```python
from build123d import *

# Parameters (mm, degrees)
ESQUISSE1_W        = 10
ESQUISSE1_H        = 3
ESQUISSE1_W_2      = 3
ESQUISSE1_H_2      = 10
BOSS_EXTRU_1_DEPTH = 3


with BuildPart() as part:
    # Esquisse1 → Boss.-Extru.1 (new body)
    with BuildSketch(Plane(origin=(0, 0, 0), x_dir=(1, 0, 0), z_dir=(0, 1, 0))):
        with BuildLine():
            Line((-48.586354215, -63.79082471), (72.626849221, -63.79082471))
            Line((72.626849221, -63.79082471), (72.626849221, -31.820261962))
            Line((72.626849221, -31.820261962), (61.846203207, -42.600907976))
            ThreePointArc((61.846203207, -42.600907976), (59.121902654, -51.239420877), (50.947990526, -47.336488751))
            Line((50.947990526, -47.336488751), (19.393465144, -47.336488751))
            Line((19.393465144, -47.336488751), (19.393465144, -44.336488751))
            Line((19.393465144, -44.336488751), (50.896342586, -44.336488751))
            ThreePointArc((50.896342586, -44.336488751), (54.339544234, -40.233556625), (59.688362254, -40.516108241))
            Line((59.688362254, -40.516108241), (72.626849221, -27.577621274))
            Line((72.626849221, -27.577621274), (72.626849221, -17.577621274))
            Line((72.626849221, -17.577621274), (-27.373150779, -17.577621274))
            Line((-27.373150779, -17.577621274), (-48.586354215, -38.79082471))
            Line((-48.586354215, -38.79082471), (-48.586354215, -63.79082471))
        make_face()
        with Locations((-1.907227595, -25.374770958)):
            Rectangle(ESQUISSE1_W, ESQUISSE1_H, mode=Mode.SUBTRACT)
        with Locations((-21.907227595, -25.374770958)):
            Rectangle(ESQUISSE1_W, ESQUISSE1_H, mode=Mode.SUBTRACT)
        with Locations((18.092772405, -25.374770958)):
            Rectangle(ESQUISSE1_W, ESQUISSE1_H, mode=Mode.SUBTRACT)
        with Locations((38.092772405, -25.374770958)):
            Rectangle(ESQUISSE1_W, ESQUISSE1_H, mode=Mode.SUBTRACT)
        with Locations((58.092772405, -25.374770958)):
            Rectangle(ESQUISSE1_W, ESQUISSE1_H, mode=Mode.SUBTRACT)
        with Locations((-21.907227595, -58.374770958)):
            Rectangle(ESQUISSE1_W, ESQUISSE1_H, mode=Mode.SUBTRACT)
        with Locations((-1.907227595, -58.374770958)):
            Rectangle(ESQUISSE1_W, ESQUISSE1_H, mode=Mode.SUBTRACT)
        with Locations((18.092772405, -58.374770958)):
            Rectangle(ESQUISSE1_W, ESQUISSE1_H, mode=Mode.SUBTRACT)
        with Locations((38.092772405, -58.374770958)):
            Rectangle(ESQUISSE1_W, ESQUISSE1_H, mode=Mode.SUBTRACT)
        with Locations((58.092772405, -58.374770958)):
            Rectangle(ESQUISSE1_W, ESQUISSE1_H, mode=Mode.SUBTRACT)
        with Locations((-25.407227595, -41.874770958)):
            Rectangle(ESQUISSE1_W_2, ESQUISSE1_H_2, mode=Mode.SUBTRACT)
    extrude(amount=BOSS_EXTRU_1_DEPTH)


solid = part.part
```
Part model, mm, in its own coordinate system. A direction names the side the tool comes from. Round coordinates to 2 decimals unless told otherwise and drop trailing zeros. Loops run counter-clockwise (first coordinate to the right, second up) from the corner with the lowest first, then second, coordinate; pieces in that order, holes last. Notation, with made-up numbers: (-33.75, 2) -> (-19.75, 2) arc R27 ccw to (-19.75, 22) -> close; hole circle Ø9 at (2, -8). An arc over 180 degrees is marked (long way). Use CSV: the item, a comma, the result in double quotes. Start each with the question number.
1) Cut at B-B, the plane z = 50.5. Write the cut outline in (x, y).
2) Wall check: L1, parallel to Z at x = 18, y = 1.65; L2, parallel to X at y = 0.7, z = 58; L3, parallel to Z at x = 40, y = 0.55. Give the ranges that are in metal, low to high. Write a range as [from, to].
3) Cut at A-A, the plane x = 15.5. Write the cut outline in (y, z).
4) Which spindle directions (+Z, -Z, +X, -X, +Y, -Y) get a long thin tool onto all of the face, cutting with end or side? Do faces 1 (the flat face through (-48.586, 1, 51)), 2 (the flat face through (18, 1, 59.875)). Say none if no direction does.
5) Cut at C-C, the plane y = 0.95. Give the number of separate pieces and of enclosed holes in the cut face, plus the area to 3 significant figures.
6) Cut at D-D, the plane x = -32. Write the cut outline in (y, z).
7) Pull direction Z, two halves, no side cores. Call faces 3 (the flat face through (-25, 1, 46.875)), 4 (the flat face through (72.627, 1, 48)), 5 (the flat face through (-22, 1, 56.875)), 6 (the flat face through (-37.831, 1.479, 28.036)): +Z half, -Z half, draft (parallel to the pull), parting line (faces both ways), or undercut.
Determined:
1,outline,"(-48.59, 0) -> (53.08, 0) -> (53.08, 3) -> (-48.59, 3) -> close; (60.38, 0) -> (72.63, 0) -> (72.63, 3) -> (60.38, 3) -> close"
2,L1,"z = [17.58, 23.87], [26.87, 56.87], [59.87, 63.79]"
2,L2,"x = [-48.59, -26.91], [-16.91, -6.91], [3.09, 13.09], [23.09, 33.09], [43.09, 53.09], [63.09, 72.63]"
2,L3,"z = [17.58, 23.87], [26.87, 44.34], [47.34, 56.87], [59.87, 63.79]"
3,outline,"(0, 17.58) -> (3, 17.58) -> (3, 23.87) -> (0, 23.87) -> close; (0, 26.87) -> (3, 26.87) -> (3, 56.87) -> (0, 56.87) -> close; (0, 59.87) -> (3, 59.87) -> (3, 63.79) -> (0, 63.79) -> close"
4,face 1,"+Z, -Z, -X, +Y, -Y"
4,face 2,"+Y, -Y"
5,separate pieces,"1"
5,enclosed holes,"11"
5,area,"4,790 mm2"
6,outline,"(0, 22.2) -> (3, 22.2) -> (3, 63.79) -> (0, 63.79) -> close"
7,face 3,"undercut"
7,face 4,"draft"
7,face 5,"undercut"
7,face 6,"-Z half"
